Geometry check sheet. Reference: the model listing, model coordinates, mm. Face numbers are marked on the shaded views. A direction names the side the tool comes from. Round coordinates to 2 decimals unless told otherwise and drop trailing zeros. Loops run counter-clockwise (first coordinate to the right, second up) from the corner with the lowest first, then second, coordinate; pieces in that order, holes last. Notation, with made-up numbers: (70.25, -1.5) -> (108.25, -1.5) arc R19 cw to (108.25, 16.5) -> close; hole circle Ø1 at (7.25, -25). An arc over 180 degrees is marked (long way). Use a Markdown table: item, result. Add a question column.
Q1. Material ranges on L1, parallel to X at y = -3.5, z = -24.5; L2, parallel to X at y = 13.5, z = -34, recorded low to high.
Q2. Set-up check for the marked faces 1, 2 and 3: record each of +Z, -Z, +X, -X, +Y, -Y from which the full face is reachable in a straight line by a thin tool's end or side.
Q3. Sectioned sample at D-D, the plane x = 1. Enter the section's corners in (y, z), then the cut area to 3 significant figures.
Q4. Gauge pin test, flat ends, axial feed: P1, Ø5, axis at y = 20, z = -13.5, coming from the -X side; P2, Ø10, axis at y = -24, z = 30, coming from the +X side; P3, Ø23, axis at y = -4, z = 17.5, coming from the -X side; P4, Ø6, axis at x = -8, y = -5.5, coming from the -Z side. Record the tip position at first contact, or that the pin passes through.
Q5. Sectioned sample at B-B, the plane z = 15. Enter the section's corners in (x, y), then the cut area to 3 significant figures.
Q6. Sectioned sample at C-C, the plane z = 0. Give the number of separate pieces and of enclosed holes in the cut face, then the cut area to 3 significant figures.
Q7. Sectioned sample at A-A, the plane y = 31.5. Enter the section's corners in (x, z).
```python
from build123d import *

# Parameters (mm, degrees)
F0_W     = 12.7
F0_H     = 38.1
F0_W_2   = 6.35
F2_R     = 9.525
F3_DEPTH = 44.45
F4_R     = 9.525
F5_DEPTH = 44.45
F6_R     = 9.525
F7_DEPTH = 44.45
F8_R     = 9.525
F9_DEPTH = 44.45


with BuildPart() as f1:
    # F0 (on Front) → F1 (revolve)
    with BuildSketch(Plane.XZ):
        Polygon((-107.95, 0), (-139.7, 0), (-139.7, -9.525), (-120.65, -9.525), (-120.65, -38.1), (-107.95, -38.1), align=None)
        with Locations((-57.15, -19.05)):
            Rectangle(F0_W, F0_H)
        with Locations((-3.175, -19.05)):
            Rectangle(F0_W_2, F0_H)
        with Locations((3.175, -19.05)):
            Rectangle(F0_W_2, F0_H)
        with Locations((57.15, -19.05)):
            Rectangle(F0_W, F0_H)
        Polygon((107.95, 0), (107.95, -38.1), (120.65, -38.1), (120.65, -9.525), (139.7, -9.525), (139.7, 0), align=None)
    revolve(axis=Axis((14.184596, 0, 0), (1, 0, 0)))

    # F2 (on face) → F3 (join, through all)
    with BuildSketch(Plane.YZ.offset(-107.95)):
        with Locations((0, -19.05)):
            Circle(F2_R)
    extrude(amount=F3_DEPTH)

    # F4 (on face) → F5 (join, through all)
    with BuildSketch(Plane.YZ.offset(-50.8)):
        with Locations((-19.05, 0)):
            Circle(F4_R)
    extrude(amount=F5_DEPTH)

    # F6 (on face) → F7 (join, through all)
    with BuildSketch(Plane.YZ.offset(6.35)):
        with Locations((0, 19.05)):
            Circle(F6_R)
    extrude(amount=F7_DEPTH)

    # F8 (on face) → F9 (join, through all)
    with BuildSketch(Plane.YZ.offset(63.5)):
        with Locations((19.05, 0)):
            Circle(F8_R)
    extrude(amount=F9_DEPTH)


solid = f1.part
```
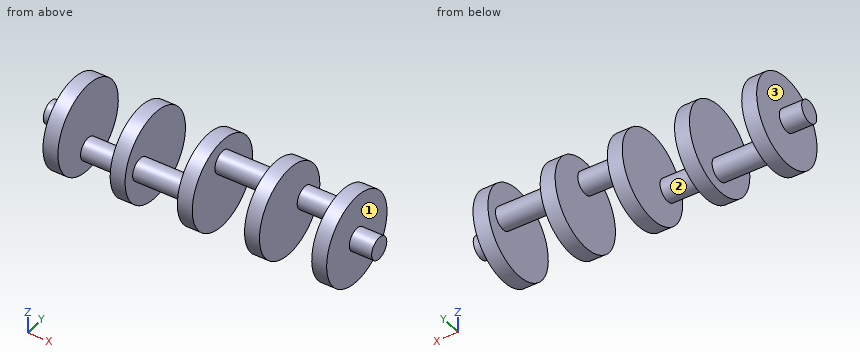
Values:
| question | item | result |
|---|---|---|
| 1 | L1 | -120.65 to -50.8, -6.35 to 6.35, 50.8 to 63.5, 107.95 to 120.65 |
| 1 | L2 | -120.65 to -107.95, -63.5 to -50.8, -6.35 to 6.35, 50.8 to 63.5, 107.95 to 120.65 |
| 2 | face 1 | +X |
| 2 | face 2 | none |
| 2 | face 3 | -X |
| 3 | outline | circle Ø76.2 at (0, 0) |
| 3 | area | 4,560 mm^2 |
| 4 | P1 | x = -120.65 |
| 4 | P2 | x = 120.65 |
| 4 | P3 | x = -139.7 |
| 4 | P4 | z = -37.98 |
| 5 | outline | (-120.65, -35.02) -> (-107.95, -35.02) -> (-107.95, 35.02) -> (-120.65, 35.02) -> close; (-63.5, -35.02) -> (-50.8, -35.02) -> (-50.8, 35.02) -> (-63.5, 35.02) -> close; (-6.35, -35.02) -> (6.35, -35.02) -> (6.35, -8.62) -> (50.8, -8.62) -> (50.8, -35.02) -> (63.5, -35.02) -> (63.5, 35.02) -> (50.8, 35.02) -> (50.8, 8.62) -> (6.35, 8.62) -> (6.35, 35.02) -> (-6.35, 35.02) -> close; (107.95, -35.02) -> (120.65, -35.02) -> (120.65, 35.02) -> (107.95, 35.02) -> close |
| 5 | area | 5,210 mm^2 |
| 6 | separate pieces | 3 |
| 6 | enclosed holes | 0 |
| 6 | area | 7,260 mm^2 |
| 7 | outline | (-120.65, -21.43) -> (-107.95, -21.43) -> (-107.95, 21.43) -> (-120.65, 21.43) -> close; (-63.5, -21.43) -> (-50.8, -21.43) -> (-50.8, 21.43) -> (-63.5, 21.43) -> close; (-6.35, -21.43) -> (6.35, -21.43) -> (6.35, 21.43) -> (-6.35, 21.43) -> close; (50.8, -21.43) -> (63.5, -21.43) -> (63.5, 21.43) -> (50.8, 21.43) -> close; (107.95, -21.43) -> (120.65, -21.43) -> (120.65, 21.43) -> (107.95, 21.43) -> close |
